Geometry check sheet. Reference: the model listing, model coordinates, mm. Face numbers are marked on the shaded views. A direction names the side the tool comes from. Round coordinates to 2 decimals unless told otherwise and drop trailing zeros. Order: outer loops, then holes, each group sorted by start corner. A loop starts at its lowest first (then second) coordinate and runs counter-clockwise, first axis right, second up.
(1) Set-up check for the marked faces 1 and 2: record each of +Z, -Z, +X, -X, +Y, -Y from which the full face is reachable in a straight line by a thin tool's end or side.
(2) Gauge pin test, flat ends, axial feed: P1, Ø8, axis at y = -2.5, z = 15.5, coming from the +X side; P2, Ø5, axis at x = 38, z = 8, coming from the +Y side; P3, Ø0.9, axis at y = -140, z = 4.5, coming from the -X side. Record the tip position at first contact, or that the pin passes through.
(3) Thickness scan on L1, parallel to Z at x = 6.5, y = -140; L2, parallel to Y at x = 90, z = 14.5. Record the ranges inside material, lowest first.
(4) Cross-section at A-A on z = 16.75. Enter the section's corners in (x, y).
(5) Cross-section at B-B on x = 77.5. Enter the section's corners in (y, z), and give its area (3 significant figures).
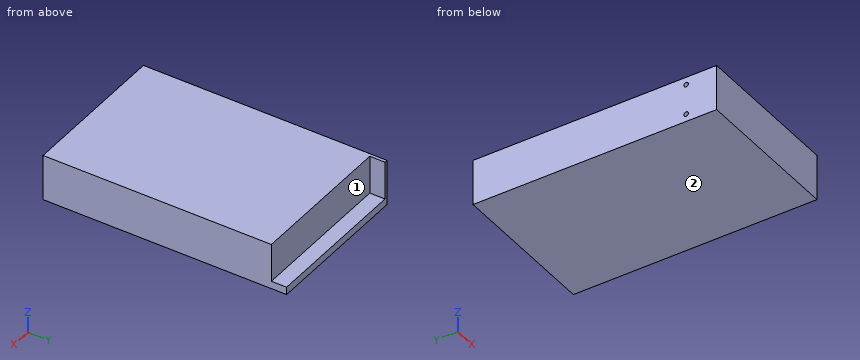
from build123d import *

# Parameters (mm, degrees)
F0_W     = 100
F0_H     = 160
F1_DEPTH = 30
F2_R     = 1.5
F3_DEPTH = 10
F4_W     = 98
F4_H     = 10
F5_DEPTH = 25


with BuildPart() as f1:
    # F0 (on Top) → F1 (new body)
    with BuildSketch(Plane.XY):
        with Locations((50, -80)):
            Rectangle(F0_W, F0_H)
    extrude(amount=F1_DEPTH)

    # F2 (on face) → F3 (cut)
    with BuildSketch(Plane(origin=(0, 0, 0), x_dir=(0, -1, 0), z_dir=(-1, 0, 0))):
        with Locations((140, 25)):
            Circle(F2_R)
        with Locations((140, 5)):
            Circle(F2_R)
    extrude(amount=-F3_DEPTH, mode=Mode.SUBTRACT)

    # F4 (on face) → F5 (cut)
    with BuildSketch(Plane.XY.offset(30)):
        with Locations((51, -5)):
            Rectangle(F4_W, F4_H)
    extrude(amount=-F5_DEPTH, mode=Mode.SUBTRACT)


solid = f1.part
Found:
1. face 1: +Z, +X, +Y
1. face 2: -Z, +X, -X, +Y, -Y
2. P1: stops at x = 2
2. P2: stops at y = -10
2. P3: stops at x = 10
3. L1: z = 0 to 3.5, 6.5 to 23.5, 26.5 to 30
3. L2: y = -160 to -10
4. outline: (0, -160) - (100, -160) - (100, -10) - (2, -10) - (2, 0) - (0, 0) - close
5. outline: (-160, 0) - (0, 0) - (0, 5) - (-10, 5) - (-10, 30) - (-160, 30) - close
5. area: 4,550 mm2
